Check sheet for the drawn part. Datum: minimum x, y, z corner. Units: mm. A direction names the side the tool comes from. Coordinates: 2 decimals unless noted, no trailing zeros. Write each loop counter-clockwise with the first axis right and the second up, starting at its lowest first coordinate (ties: lowest second). Pieces come first, ordered by that corner, then holes. Notation, with made-up numbers: (-18, 73.25) -> (4, 73.25) arc R31 cw to (4, 107.25) -> close; hole circle Ø11 at (-8.5, -6). An arc over 180 degrees is marked (long way). Write item = value, one per line. Start each with the question number.
(1) Section check A-A (x = 39). Record the cut outline in (y, z), plus the area to 3 significant figures.
(2) Material ranges on probe 1 along Z at (x, y) = (45.5, 12.5); probe 2 along Y at (x, z) = (4.5, 25), recorded low to high. Write a range as [from, to].
(3) Set-up check for the marked faces 5 and 6: record each of +Z, -Z, +X, -X, +Y, -Y from which the full face is reachable in a straight line by a thin tool's end or side.
(4) Section check B-B (y = 19). Record the cut outline in (x, z).
(5) Gauge pin test, flat ends, axial feed: pin 1 Ø10 at (y, z) = (35.5, 50.5) entering from -X; pin 2 Ø2 at (y, z) = (6, 1) entering from -X; pin 3 Ø3 at (y, z) = (9, 79) entering from +X; pin 4 Ø10 at (x, z) = (28, 49) entering from -Y. Record the tip position at first contact, or that the pin passes through.
(6) Section check C-C (z = 31). Record the cut outline in (x, y).
(7) Mould release check, pull along Z, two halves, no side actions. Record for the marked faces 1, 2, 3 and 4: released by +Z, released by -Z, zero draft, split by the parting line, or undercut.
(8) Section check D-D (x = 30). Record the cut outline in (y, z).
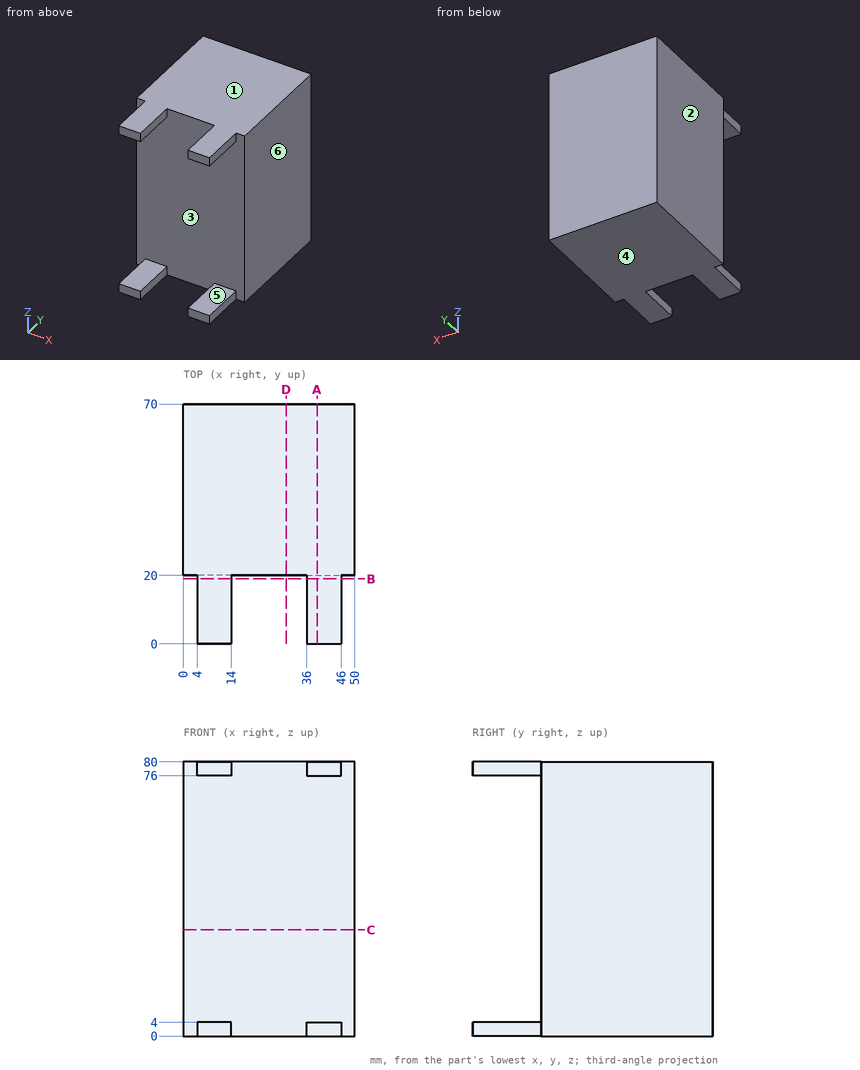
Response:
q1.outline = (0, 0) -> (70, 0) -> (70, 80) -> (0, 80) -> (0, 76) -> (20, 76) -> (20, 4) -> (0, 4) -> close
q1.area = 4,160 mm2
q2.probe_1 = [0, 4], [76, 80]
q2.probe_2 = [20, 70]
q3.face_5 = +X, -X, -Y
q3.face_6 = +Z, -Z, +X, +Y, -Y
q4.outline = (4, 0) -> (14, 0) -> (14, 4) -> (4, 4) -> close; (4, 76) -> (14, 76) -> (14, 80) -> (4, 80) -> close; (36, 0) -> (46, 0) -> (46, 4) -> (36, 4) -> close; (36, 76) -> (46, 76) -> (46, 80) -> (36, 80) -> close
q5.pin_1 = 0
q5.pin_2 = 4
q5.pin_3 = 46
q5.pin_4 = 20
q6.outline = (0, 20) -> (50, 20) -> (50, 70) -> (0, 70) -> close
q7.face_1 = released by +Z
q7.face_2 = zero draft
q7.face_3 = undercut
q7.face_4 = released by -Z
q8.outline = (20, 0) -> (70, 0) -> (70, 80) -> (20, 80) -> close
